Design review of the part built by this model. Coordinates are the model's own, in mm. A direction names the side the tool comes from. Give positions to 0.01 mm unless a question says otherwise; leave off trailing zeros. Write each loop counter-clockwise with the first axis right and the second up, starting at its lowest first coordinate (ties: lowest second). Pieces come first, ordered by that corner, then holes. Notation, with made-up numbers: M 49.25,55 L 70.25,55 A32 cw 70.25,94 Z; hole C 4,75 d2. An arc over 180 degrees is marked long. Use a Markdown table: item, result. Add a question column.
```python
from build123d import *

# Parameters (mm, degrees)
SKETCH1_R            = 4
SKETCH1_R_2          = 2
BOSS_EXTRUDE1_DEPTH  = 2
CUT_SWEEP2_PROFILE_R = 1.5
CHAMFER1_SIZE        = 1.5


with BuildPart() as part:
    # Sketch1 → Boss-Extrude1 (new body)
    with BuildSketch(Plane.XY):
        with BuildLine():
            Line((-13, 8.952546351), (-13, 4.3251588))
            ThreePointArc((-13, 4.3251588), (-12.595694104, 3.119438963), (-11.546239674, 2.401198764))
            Line((-11.546239674, 2.401198764), (8.453760326, -3.277086269))
            ThreePointArc((8.453760326, -3.277086269), (10.205719837, -2.948820337), (11, -1.353126233))
            Line((11, -1.353126233), (11, 4.5))
            ThreePointArc((11, 4.5), (8.803300859, 9.803300859), (3.5, 12))
            Line((3.5, 12), (-7.759513818, 12))
            ThreePointArc((-7.759513818, 12), (-9.900828742, 11.687820977), (-11.86388404, 10.777272105))
            Line((-11.86388404, 10.777272105), (-12.094498726, 10.626485579))
            ThreePointArc((-12.094498726, 10.626485579), (-12.759118736, 9.904124658), (-13, 8.952546351))
        make_face()
        with Locations((4, 5)):
            Circle(SKETCH1_R, mode=Mode.SUBTRACT)
        with Locations((-9, 8.2)):
            Circle(SKETCH1_R_2, mode=Mode.SUBTRACT)
    extrude(amount=BOSS_EXTRUDE1_DEPTH)

    # Cut-Sweep2: sweep along a path in Sketch19
    with BuildLine(Plane.XY.offset(3)) as cut_sweep2_path:
        Line((-1, -3.013992868), (-1, 5))
        ThreePointArc((-1, 5), (4, 10), (9, 5))
        Line((9, 5), (9, -6.134852042))
    # Cut-Sweep2 profile (on start of the path) → Cut-Sweep2 (sweep, cut)
    with BuildSketch(Plane(origin=(-1, -3.013992868, 3), x_dir=(0, 0, 1), z_dir=(0, 1, 0))):
        Circle(CUT_SWEEP2_PROFILE_R)
    sweep(path=cut_sweep2_path.line, mode=Mode.SUBTRACT)

    # Chamfer1
    chamfer1_edges = [part.edges().sort_by_distance(p)[0] for p in [
        (-11, 8.2, 0),
    ]]
    chamfer(chamfer1_edges, length=CHAMFER1_SIZE)


solid = part.part
```
(1) Add section D-D on x = 4. Give the boundary of the cut face in (y, z), then the cut area to 3 significant figures.
(2) Machinability: for faces 1 (the flat face through (-5, 7, 2)), 2 (the cylindrical face through (-1, 2.1, 1.5)), which of the approach directions +Z, -Z, +X, -X, +Y, -Y give a long, thin tool a straight path to every point of the face, cutting with its end or side? Answer none if there is none.
(3) Add section A-A on x = -9. Give the boundary of the cut face in (y, z).
(4) Wall thickness on L1, parallel to Y at x = 4.75, z = 1.7 (3 decimals); L2, parallel to X at y = 6.5, z = 1.05; L3, parallel to Y at x = 4.75, z = 0.9: over which ranges is each line inside the solid? List them lowest first.
(5) The part is to be moulded in two halves that separate along X. For faces 3 (the cylindrical face through (3.133, 1.095, 0.986)), 4 (the flat face through (-2, 12, 1)), 5 (the cylindrical face through (-9.872, 11.696, 0.986)), say which applies: released by +X, released by -X, zero draft, split by the parting line, or undercut.
(6) Add section C-C on y = 0.25. Give the boundary of the cut face in (x, z), then the cut area to 3 significant figures.
(7) Add section B-B on z = 1. Give the boundary of the cut face in (x, y).
From the geometry:
| question | item | result |
|---|---|---|
| 1 | outline | M -2.01,0 L 1,0 L 1,2 L -2.01,2 Z; M 9,0 L 11.98,0 L 11.98,2 L 11.12,2 A1.5 cw 9,1.88 Z |
| 1 | area | 11.2 mm^2 |
| 2 | face 1 | +Z, +X, -X, +Y, -Y |
| 2 | face 2 | +Z, -Y |
| 3 | outline | M 1.68,0 L 4.7,0 L 6.2,1.5 L 6.2,2 L 1.68,2 Z; M 10.2,1.5 L 11.7,0 L 11.9,0 L 11.9,2 L 10.2,2 Z |
| 4 | L1 | y = -2.226 to 1.071, 8.929 to 9.185, 10.699 to 11.895 |
| 4 | L2 | x = -13 to -10.76, -7.24 to 0.29, 7.71 to 10.73 |
| 4 | L3 | y = -2.23 to 1.07, 8.93 to 11.9 |
| 5 | face 3 | undercut |
| 5 | face 4 | zero draft |
| 5 | face 5 | released by -X |
| 6 | outline | M -3.97,0 L 11,0 L 11,2 L 10.12,2 A1.5 cw 7.88,2 L 0.12,2 A1.5 cw -2.12,2 L -3.97,2 Z |
| 6 | area | 28.4 mm^2 |
| 7 | outline | M -13,4.33 A2 ccw -11.55,2.4 L 8.45,-3.28 A2 ccw 11,-1.35 L 11,4.5 A7.5 ccw 3.5,12 L -7.76,12 A7.5 ccw -11.86,10.78 L -12.09,10.63 A2 ccw -13,8.95 Z; hole C -9,8.2 d5; hole C 4,5 d8 |
